Read the model definition and answer for the solid it produces. Units are mm, in the model's axes. Round coordinates to 2 decimals unless told otherwise and drop trailing zeros. Write each loop counter-clockwise with the first axis right and the second up, starting at its lowest first coordinate (ties: lowest second). Pieces come first, ordered by that corner, then holes. Notation, with made-up numbers: (10.25, 36.25) - (19.25, 36.25) arc R19 ccw to (19.25, 69.25) - close; hole circle Ø4 at (-30, -18). An arc over 180 degrees is marked (long way). Answer as CSV lines item,"result". Start each with the question number.
1) Find section A-A on z = 0. Determine the outline of the cut face in (x, y).
2) Consider line 1 along X through (y, z) = (-1.25, -7); line 2 along X through (y, z) = (-3.75, 3.75); line 3 along Z through (x, y) = (298.5, 6.75). Determine where each line is inside the solid, lowest interval first.
3) Each of these flat-tipped pins is pushed along its axis until it touches: pin 1 (1 mm diameter, centred on y = 5.5, z = 6, fed in from +X); pin 2 (4 mm diameter, centred on x = 554, y = -7, fed in from -Z); pin 3 (2 mm diameter, centred on x = 416.5, z = -7, fed in from -Y). Where does it stop, or does it pass through?
4) Find section C-C on x = 633. Determine the outline of the cut face in (y, z), then the cut area to 3 significant figures.
from build123d import *

# Parameters (mm, degrees)
SKETCH_W      = 700
SKETCH_H      = 10
SKETCH001_W   = 67
SKETCH001_H   = 2.5
SKETCH002_W   = 20
SKETCH002_H   = 1.5
SKETCH003_W   = 13
SKETCH003_H   = 2.5
SKETCH003_W_2 = 1
SKETCH003_H_2 = 3.01


with BuildPart() as part:
    # Sketch → Revolution (revolve)
    with BuildSketch(Plane.XZ):
        with Locations((350, 5)):
            Rectangle(SKETCH_W, SKETCH_H)
    revolve(axis=Axis((0, 0, 0), (1, 0, 0)))

    # Sketch001 → Groove (revolve, cut)
    with BuildSketch(Plane.XZ):
        with Locations((33.5, 8.75)):
            Rectangle(SKETCH001_W, SKETCH001_H)
    revolve(axis=Axis((0, 0, 0), (1, 0, 0)), mode=Mode.SUBTRACT)

    # Sketch002 → Groove001 (revolve, cut)
    with BuildSketch(Plane.XZ):
        with Locations((10, 6.75)):
            Rectangle(SKETCH002_W, SKETCH002_H)
    revolve(axis=Axis((0, 0, 0), (1, 0, 0)), mode=Mode.SUBTRACT)

    # Sketch003 → Groove002 (revolve, cut)
    with BuildSketch(Plane.XZ):
        with Locations((693.5, 8.75)):
            Rectangle(SKETCH003_W, SKETCH003_H)
        with Locations((696.5, 5.995)):
            Rectangle(SKETCH003_W_2, SKETCH003_H_2)
    revolve(axis=Axis((0, 0, 0), (1, 0, 0)), mode=Mode.SUBTRACT)


solid = part.part
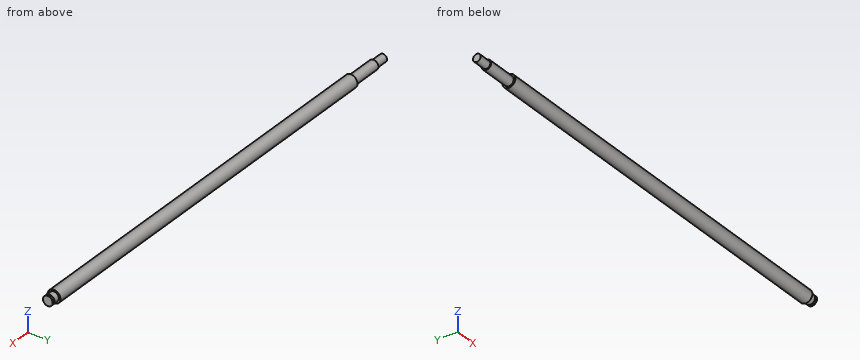
Check values:
1,outline,"(0, -6) - (20, -6) - (20, -7.5) - (67, -7.5) - (67, -10) - (687, -10) - (687, -7.5) - (696, -7.5) - (696, -4.49) - (697, -4.49) - (697, -7.5) - (700, -7.5) - (700, 7.5) - (697, 7.5) - (697, 4.49) - (696, 4.49) - (696, 7.5) - (687, 7.5) - (687, 10) - (67, 10) - (67, 7.5) - (20, 7.5) - (20, 6) - (0, 6) - close"
2,line 1,"x = 20 to 696, 697 to 700"
2,line 2,"x = 0 to 696, 697 to 700"
2,line 3,"z = -7.38 to 7.38"
3,pin 1,"stops at x = 687"
3,pin 2,"stops at z = -8.66"
3,pin 3,"stops at y = -8"
4,outline,"circle Ø20 at (0, 0)"
4,area,"314 mm^2"
